from build123d import *

# Parameters (mm, degrees)
F0_W     = 57.15
F0_H     = 38.1
F1_DEPTH = 28.829
F2_W     = 18.8468
F2_H     = 9.525
F3_DEPTH = 38.101
F4_W     = 18.8468
F4_H     = 18.542
F5_DEPTH = 9.652


with BuildPart() as f1:
    # F0 (on Top) → F1 (new body)
    with BuildSketch(Plane.XY):
        with Locations((-28.575, -0.834305)):
            Rectangle(F0_W, F0_H)
    extrude(amount=F1_DEPTH)

    # F2 (on face) → F3 (cut, through all)
    with BuildSketch(Plane.XZ.offset(19.884305)):
        Polygon((-57.15, 28.829), (-57.15, 9.652), (-38.1, 9.652), (-38.1, 19.2405), (-38.1, 19.304), (-38.1, 28.829), align=None)
        with Locations((-28.6766, 24.0665)):
            Rectangle(F2_W, F2_H)
    extrude(amount=-F3_DEPTH, mode=Mode.SUBTRACT)

    # F4 (on face) → F5 (cut)
    with BuildSketch(Plane.XY.offset(19.304)):
        with Locations((-28.6766, -0.834305)):
            Rectangle(F4_W, F4_H)
    extrude(amount=-F5_DEPTH, mode=Mode.SUBTRACT)


solid = f1.part
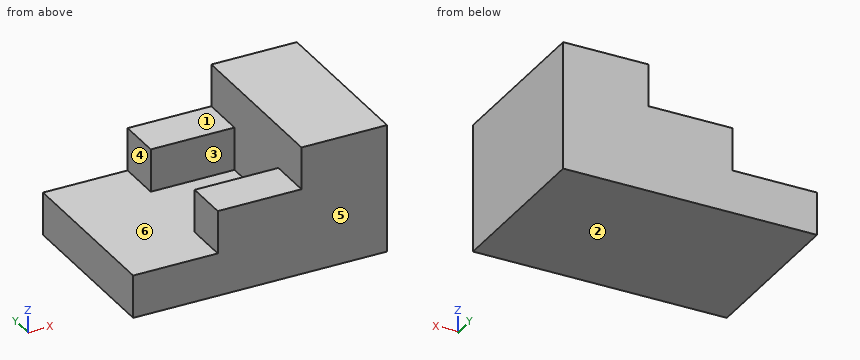
Work out the finished part from the listing and answer in its coordinate system (mm). Face numbers are marked on the shaded views. A direction names the side the tool comes from. Round coordinates to 2 decimals unless told otherwise and drop trailing zeros. Write each loop counter-clockwise with the first axis right and the second up, starting at its lowest first coordinate (ties: lowest second). Pieces come first, ordered by that corner, then holes. Notation, with made-up numbers: (39.25, 9.5) - (90.25, 9.5) arc R19 ccw to (90.25, 24.5) - close; hole circle Ø2 at (-8.75, -36.5). An arc over 180 degrees is marked (long way). Answer in a Markdown table with one row per item. Add a question column.
1. Find the intervals of material crossed by line 1 along X through (y, z) = (11.5, 20.25); line 2 along Z through (x, y) = (-40, 6.5); line 3 along X through (y, z) = (9, 18), in increasing order. Write a range as from..to.
2. For the marked faces 1, 2 and 3, determine the directions among +Z, -Z, +X, -X, +Y, -Y from which every point of the face is accessible in a straight line to the end or side of a thin tool.
3. Given pin 1 (8 mm diameter, centred on y = -3.5, z = 24, fed in from -X); pin 2 (5 mm diameter, centred on y = -15.5, z = 14, fed in from -X); pin 3 (3 mm diameter, centred on x = -26, y = 11, fed in from +Z), each flat-ended and moving along its own axis, determine where each tip first touches the part or whether it passes through.
4. A cutting plane is placed at A-A, the plane z = 16. Determine the outline of the cut face in (x, y).
5. A cutting plane is placed at B-B, the plane y = -15.5. Determine the outline of the cut face in (x, z), and give its area (3 significant figures).
6. The mould has two halves that part along Y. Classify the marked faces 4, 5 and 6: +Y half, -Y half, draft (parallel to the pull), parting line (faces both ways), or undercut.
7. A cutting plane is placed at C-C, the plane x = -39. Determine the outline of the cut face in (y, z).
8. A cutting plane is placed at D-D, the plane y = 3. Determine the outline of the cut face in (x, z), and give its area (3 significant figures).
Worked out:
| question | item | result |
|---|---|---|
| 1 | line 1 | -19.25..0 |
| 1 | line 2 | 0..9.65 |
| 1 | line 3 | -38.1..0 |
| 2 | face 1 | +Z, -X, +Y, -Y |
| 2 | face 2 | -Z, +X, -X, +Y, -Y |
| 2 | face 3 | +Z, -X |
| 3 | pin 1 | x = -19.25 |
| 3 | pin 2 | x = -38.1 |
| 3 | pin 3 | z = 19.3 |
| 4 | outline | (-38.1, -19.88) - (0, -19.88) - (0, 18.22) - (-38.1, 18.22) - (-38.1, 8.44) - (-19.25, 8.44) - (-19.25, -10.11) - (-38.1, -10.11) - close |
| 5 | outline | (-57.15, 0) - (0, 0) - (0, 28.83) - (-19.25, 28.83) - (-19.25, 19.3) - (-38.1, 19.3) - (-38.1, 9.65) - (-57.15, 9.65) - close |
| 5 | area | 1,100 mm^2 |
| 6 | face 4 | draft |
| 6 | face 5 | -Y half |
| 6 | face 6 | undercut |
| 7 | outline | (-19.88, 0) - (18.22, 0) - (18.22, 9.65) - (-19.88, 9.65) - close |
| 8 | outline | (-57.15, 0) - (0, 0) - (0, 28.83) - (-19.25, 28.83) - (-19.25, 9.65) - (-57.15, 9.65) - close |
| 8 | area | 921 mm^2 |
